Verification items for the finished model (mm, model axes). Face numbers are marked on the shaded views. A direction names the side the tool comes from. Coordinates: 2 decimals unless noted, no trailing zeros. Order: outer loops, then holes, each group sorted by start corner. A loop starts at its lowest first (then second) coordinate and runs counter-clockwise, first axis right, second up. Notation, with made-up numbers: M 64,-10.75 L 104,-10.75 A19 ccw 104,25.25 Z; hole C 37.5,4 d11. An arc over 180 degrees is marked long. Write item = value, one per line.
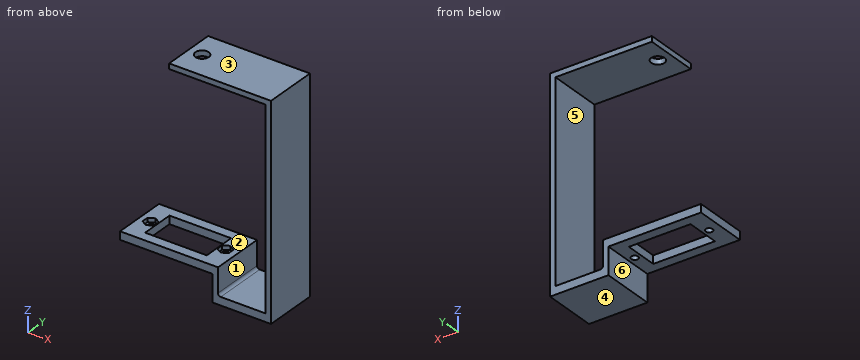
```python
from build123d import *

# Parameters (mm, degrees)
BOSS_EXTRUDE1_START       = 26.09
SKETCH2_W                 = 20
SKETCH2_H                 = 73
BOSS_EXTRUDE1_DEPTH       = 2
SKETCH3_W                 = 37.815629263
SKETCH3_H                 = 20
SKETCH3_R                 = 2.5
BOSS_EXTRUDE2_DEPTH       = 2
BOSS_EXTRUDE3_START       = -3
BOSS_EXTRUDE3_OUTLINE_W   = 34.391343997
BOSS_EXTRUDE3_OUTLINE_H   = 20
BOSS_EXTRUDE3_OUTLINE_R   = 1.1
BOSS_EXTRUDE3_OUTLINE_W_2 = 22.89999
BOSS_EXTRUDE3_OUTLINE_H_2 = 12.5
BOSS_EXTRUDE3_DEPTH       = 3
SKETCH7_W                 = 10
SKETCH7_H                 = 20
BOSS_EXTRUDE4_DEPTH       = 2
SKETCH8_W                 = 21.665624263
SKETCH8_H                 = 20
BOSS_EXTRUDE5_DEPTH       = 3
FILLET1_R                 = 1
CUT_EXTRUDE5_START        = -3
SKETCH4_3_R               = 1.1
CUT_EXTRUDE5_DEPTH        = 1.5
M2_CLEARANCE_HOLE1_D      = 2.6
M2_CLEARANCE_HOLE1_DEPTH  = 3
M2_CLEARANCE_HOLE1_TIP    = 0.781118805


# Read off the part's stored shape, not the designer's step: Boss-Extrude3
with BuildPart() as part:
    # Sketch2 → Boss-Extrude1 (new body)
    with BuildSketch(Plane(origin=(0, 0, 13.2), x_dir=(0, 1, 0), z_dir=(1, 0, 0)).offset(BOSS_EXTRUDE1_START)):
        with Locations((-24.849481376, -4.332139258)):
            Rectangle(SKETCH2_W, SKETCH2_H)
    extrude(amount=BOSS_EXTRUDE1_DEPTH)

    # Sketch3 → Boss-Extrude2 (add)
    with BuildSketch(Plane.XY.offset(45.367860742)):
        with Locations((9.182185369, -24.849481376)):
            Rectangle(SKETCH3_W, SKETCH3_H)
        with Locations((-4.725629263, -24.849481376)):
            Circle(SKETCH3_R, mode=Mode.SUBTRACT)
    extrude(amount=BOSS_EXTRUDE2_DEPTH)



with BuildPart() as body_2:
    # Boss-Extrude3 outline → Boss-Extrude3 (new body)
    with BuildSketch(Plane(origin=(0, 0, -20.632139258), x_dir=(-1, 0, 0), z_dir=(0, 0, -1)).offset(BOSS_EXTRUDE3_START)):
        with Locations((10.771296262, -24.849481376)):
            Rectangle(BOSS_EXTRUDE3_OUTLINE_W, BOSS_EXTRUDE3_OUTLINE_H)
        with Locations((-3.924375737, -24.849481376)):
            Circle(BOSS_EXTRUDE3_OUTLINE_R, mode=Mode.SUBTRACT)
        with Locations((9.925624263, -24.849481376)):
            Rectangle(BOSS_EXTRUDE3_OUTLINE_W_2, BOSS_EXTRUDE3_OUTLINE_H_2, mode=Mode.SUBTRACT)
        with Locations((23.775624263, -24.849481376)):
            Circle(BOSS_EXTRUDE3_OUTLINE_R, mode=Mode.SUBTRACT)
    extrude(amount=BOSS_EXTRUDE3_DEPTH)

    # Sketch7 → Boss-Extrude4 (add)
    with BuildSketch(Plane(origin=(6.424375737, 0, 0), x_dir=(0, 0, -1), z_dir=(1, 0, 0))):
        with Locations((22.632139258, -24.849481376)):
            Rectangle(SKETCH7_W, SKETCH7_H)
    extrude(amount=BOSS_EXTRUDE4_DEPTH)


with BuildPart() as part_1:
    add(part.part)

    add(body_2.part)  # Boss-Extrude5 merges body 2
    # Sketch8 → Boss-Extrude5 (add)
    with BuildSketch(Plane(origin=(0, 0, -27.632139258), x_dir=(-1, 0, 0), z_dir=(0, 0, -1))):
        with Locations((-17.257187869, -24.849481376)):
            Rectangle(SKETCH8_W, SKETCH8_H)
    extrude(amount=BOSS_EXTRUDE5_DEPTH)

    # Fillet1
    fillet1_edges = [part_1.edges().sort_by_distance(p)[0] for p in [
        (8.424375737, -24.849481376, -27.632139258),
    ]]
    fillet(fillet1_edges, radius=FILLET1_R)

    # Sketch4<3> → Cut-Extrude5 (cut)
    # profile 1 of 4: a face of its own
    with BuildSketch(Plane(origin=(0, 0, -20.632139258), x_dir=(-1, 0, 0), z_dir=(0, 0, -1)).offset(CUT_EXTRUDE5_START)):
        Polygon((-3.965719734, -22.379328504), (-1.815719734, -23.620631583), (-1.815719734, -26.103237741), (-3.965719734, -27.344540819), (-6.115719734, -26.103237741), (-6.115719734, -23.620631583), align=None)
        with Locations((-3.924375737, -24.849481376)):
            Circle(SKETCH4_3_R, mode=Mode.SUBTRACT)
    # profile 2 of 4: a face of its own
    with BuildSketch(Plane(origin=(0, 0, -20.632139258), x_dir=(-1, 0, 0), z_dir=(0, 0, -1)).offset(CUT_EXTRUDE5_START)):
        Polygon((23.81696826, -22.379328504), (21.66696826, -23.620631583), (21.66696826, -26.103237741), (23.81696826, -27.344540819), (25.96696826, -26.103237741), (25.96696826, -23.620631583), align=None)
        with Locations(Location((23.775624263, -24.849481376, 0), (0, 0, 180))):
            Circle(SKETCH4_3_R, mode=Mode.SUBTRACT)
    # profile 3 of 4: a face of its own
    with BuildSketch(Plane(origin=(0, 0, -20.632139258), x_dir=(-1, 0, 0), z_dir=(0, 0, -1)).offset(CUT_EXTRUDE5_START)):
        with Locations((-3.924375737, -24.849481376)):
            Circle(SKETCH4_3_R)
    # profile 4 of 4: a face of its own
    with BuildSketch(Plane(origin=(0, 0, -20.632139258), x_dir=(-1, 0, 0), z_dir=(0, 0, -1)).offset(CUT_EXTRUDE5_START)):
        with Locations(Location((23.775624263, -24.849481376, 0), (0, 0, 180))):
            Circle(SKETCH4_3_R)
    extrude(amount=CUT_EXTRUDE5_DEPTH, mode=Mode.SUBTRACT)

    # M2 Clearance Hole1
    with Locations(Plane(origin=(0, 0, -20.632139258), x_dir=(-1, 0, 0), z_dir=(0, 0, -1))):
        with Locations((-3.924375737, -24.849481376), (23.775624263, -24.849481376)):
            Hole(M2_CLEARANCE_HOLE1_D / 2, depth=M2_CLEARANCE_HOLE1_DEPTH)
            with Locations((0, 0, -(M2_CLEARANCE_HOLE1_DEPTH + M2_CLEARANCE_HOLE1_TIP / 2))):  # 118° drill point
                Cone(0, M2_CLEARANCE_HOLE1_D / 2, M2_CLEARANCE_HOLE1_TIP, mode=Mode.SUBTRACT)


solid = part_1.part
```
Item 1: Tool access check on the marked faces 1, 2 and 3. Record the directions out of +Z, -Z, +X, -X, +Y, -Y that give a thin tool (end or side, any length) a straight path to the whole face; none if there is none.
Report:
face_1 = +Y, -Y
face_2 = -X, +Y, -Y
face_3 = +Z, +X, -X, +Y, -Y
Item 2: Release check for a two-part mould opening along Z. For the marked faces 4, 5 and 6 record: pulls with the +Z half, pulls with the -Z half, needs draft (parallel to the pull), parting line crosses it, or undercut.
Report:
face_4 = pulls with the -Z half
face_5 = undercut
face_6 = needs draft
Item 3: Sectioned sample at D-D, the plane x = 17. Enter the section's corners in (y, z), then the cut area to 3 significant figures.
Report:
outline = M -34.85,-30.63 L -14.85,-30.63 L -14.85,-27.63 L -34.85,-27.63 Z; M -34.85,45.37 L -14.85,45.37 L -14.85,47.37 L -34.85,47.37 Z
area = 100 mm^2
Item 4: Scan lines: L1, parallel to Z at x = 11, y = -21; L2, parallel to X at y = -33.5, z = -22; L3, parallel to Z at x = 6, y = -31. Record each from-to range of solid material in increasing order. Write a range as from..to.
Report:
L1 = -30.63..-27.63, 45.37..47.37
L2 = 6.42..8.42, 26.09..28.09
L3 = -20.63..-17.63, 45.37..47.37
Item 5: Gauge pin test, flat ends, axial feed: pin 1 (2 mm diameter, centred on x = -24.5, y = -24.5, fed in from +Z); pin 2 (3 mm diameter, centred on x = -17, y = -33, fed in from +Z); pin 3 (1.5 mm diameter, centred on y = -18, z = 33, fed in from -X); pin 4 (2 mm diameter, centred on x = -23.78, y = -24.85, fed in from +Z). Record the tip position at first contact, or that the pin passes through.
Report:
pin_1 = -19.13
pin_2 = -17.63
pin_3 = 26.09
pin_4 = through
Item 6: Sectioned sample at B-B, the plane y = -28.75. Enter the section's corners in (x, z).
Report:
outline = M -27.97,-20.63 L -21.38,-20.63 L -21.38,-17.63 L -27.97,-17.63 Z; M -9.73,45.37 L 26.09,45.37 L 26.09,-27.63 L 9.42,-27.63 A1 cw 8.42,-26.63 L 8.42,-17.63 L 1.52,-17.63 L 1.52,-20.63 L 6.42,-20.63 L 6.42,-30.63 L 28.09,-30.63 L 28.09,47.37 L -9.73,47.37 Z
Item 7: Sectioned sample at A-A, the plane x = -1. Enter the section's corners in (y, z), then the cut area to 3 significant figures.
Report:
outline = M -34.85,-20.63 L -31.1,-20.63 L -31.1,-17.63 L -34.85,-17.63 Z; M -34.85,45.37 L -14.85,45.37 L -14.85,47.37 L -34.85,47.37 Z; M -18.6,-20.63 L -14.85,-20.63 L -14.85,-17.63 L -18.6,-17.63 Z
area = 62.5 mm^2
Item 8: Sectioned sample at C-C, the plane z = -25. Enter the section's corners in (x, y).
Report:
outline = M 6.42,-34.85 L 8.42,-34.85 L 8.42,-14.85 L 6.42,-14.85 Z; M 26.09,-34.85 L 28.09,-34.85 L 28.09,-14.85 L 26.09,-14.85 Z
